Read the model definition and answer for the solid it produces. Units are mm, in the model's axes. Coordinates: 2 decimals unless noted, no trailing zeros. Loops run counter-clockwise (first coordinate to the right, second up) from the corner with the lowest first, then second, coordinate; pieces in that order, holes last.
Q1. Section B-B (y = -0.6) is taken. Count the separate pieces of the cut face and the enclosed holes in it, then the cut area to 3 significant figures.
Q2. Straight lines are drawn through the part: line 1 (X direction, y = -0.55, z = -16.29); line 2 (Z direction, x = -27.62, y = -0.35); line 3 (X direction, y = -1.2, z = 3). For each, find the intervals that lie inside material, in ascending order.
Q3. Section C-C (z = -4) is taken. Give the vertices of the cut face in (x, y), then the cut area to 3 significant figures.
Q4. Section A-A (z = 16.29) is taken. Give the vertices of the cut face in (x, y).
from build123d import *

# Parameters (mm, degrees)
SKETCH1_R           = 0.2999994
SKETCH1_R_2         = 1.1
SKETCH1_R_3         = 0.499999
SKETCH1_R_4         = 0.3999992
BOSS_EXTRUDE1_DEPTH = 1.6


with BuildPart() as part:
    # Sketch1 → Boss-Extrude1 (new body)
    with BuildSketch(Plane(origin=(0, 0, 0), x_dir=(1, 0, 0), z_dir=(0, 1, 0))):
        with BuildLine():
            Line((34, -18), (34, -7.5))
            Line((34, -7.5), (30, -7.5))
            Line((30, -7.5), (30, 7.5))
            Line((30, 7.5), (34, 7.5))
            Line((34, 7.5), (34, 18))
            ThreePointArc((34, 18), (33.707106781, 18.707106781), (33, 19))
            Line((33, 19), (-29, 19))
            ThreePointArc((-29, 19), (-29.707106781, 18.707106781), (-30, 18))
            Line((-30, 18), (-30, -18))
            ThreePointArc((-30, -18), (-29.707106781, -18.707106781), (-29, -19))
            Line((-29, -19), (33, -19))
            ThreePointArc((33, -19), (33.707106781, -18.707106781), (34, -18))
        make_face()
        with Locations(Location((27.62000064, 13.199999, 0), (0, 0, 90))):
            Circle(SKETCH1_R, mode=Mode.SUBTRACT)
        with Locations(Location((27.28999876, -16.29000044, 0), (0, 0, 90))):
            Circle(SKETCH1_R_2, mode=Mode.SUBTRACT)
        with Locations(Location((27.62000064, -13.199999, 0), (0, 0, 90))):
            Circle(SKETCH1_R, mode=Mode.SUBTRACT)
        with Locations(Location((14.65628514, 14.92444056, 0), (0, 0, 90))):
            Circle(SKETCH1_R_3, mode=Mode.SUBTRACT)
        with Locations(Location((27.28999876, 16.29000044, 0), (0, 0, 90))):
            Circle(SKETCH1_R_2, mode=Mode.SUBTRACT)
        with Locations(Location((6.6676143, 14.9207728, 0), (0, 0, 90))):
            Circle(SKETCH1_R_3, mode=Mode.SUBTRACT)
        with Locations(Location((-23.75582498, 15.12569238, 0), (0, 0, 90))):
            Circle(SKETCH1_R_3, mode=Mode.SUBTRACT)
        with Locations(Location((-26.84364202, 8.59971356, 0), (0, 0, 90))):
            Circle(SKETCH1_R_4, mode=Mode.SUBTRACT)
        with Locations(Location((-27.28999876, -16.29000044, 0), (0, 0, 90))):
            Circle(SKETCH1_R_2, mode=Mode.SUBTRACT)
        with Locations(Location((-27.62000064, -13.199999, 0), (0, 0, 90))):
            Circle(SKETCH1_R, mode=Mode.SUBTRACT)
        with Locations(Location((-26.84364202, 10.8197142, 0), (0, 0, 90))):
            Circle(SKETCH1_R_4, mode=Mode.SUBTRACT)
        with Locations(Location((-23.75582498, 17.66569238, 0), (0, 0, 90))):
            Circle(SKETCH1_R_3, mode=Mode.SUBTRACT)
        with Locations(Location((-27.62000064, 13.199999, 0), (0, 0, 90))):
            Circle(SKETCH1_R, mode=Mode.SUBTRACT)
        with Locations(Location((-27.28999876, 16.29000044, 0), (0, 0, 90))):
            Circle(SKETCH1_R_2, mode=Mode.SUBTRACT)
    extrude(amount=-BOSS_EXTRUDE1_DEPTH)


solid = part.part
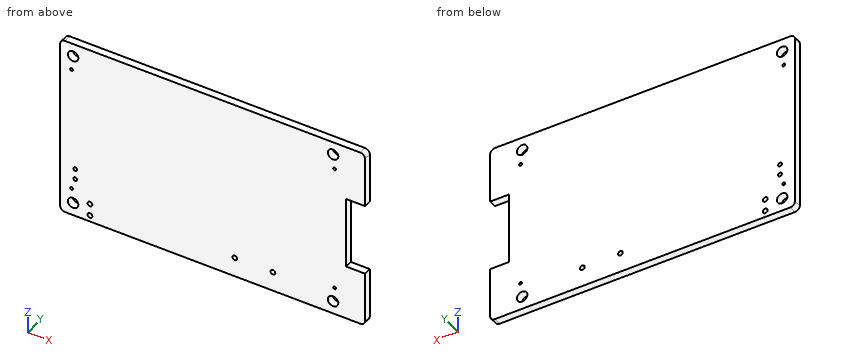
Numbers:
1. separate pieces: 1
1. enclosed holes: 14
1. area: 2,350 mm2
2. line 1: x = -30 to -28.39, -26.19 to 26.19, 28.39 to 34
2. line 2: z = -19 to -17.34, -15.24 to -13.5, -12.9 to 12.9, 13.5 to 15.24, 17.34 to 19
2. line 3: x = -30 to 30
3. outline: (-30, -1.6) - (30, -1.6) - (30, 0) - (-30, 0) - close
3. area: 96.0 mm2
4. outline: (-30, -1.6) - (-28.39, -1.6) - (-28.39, 0) - (-30, 0) - close; (-26.19, -1.6) - (26.19, -1.6) - (26.19, 0) - (-26.19, 0) - close; (28.39, -1.6) - (34, -1.6) - (34, 0) - (28.39, 0) - close
